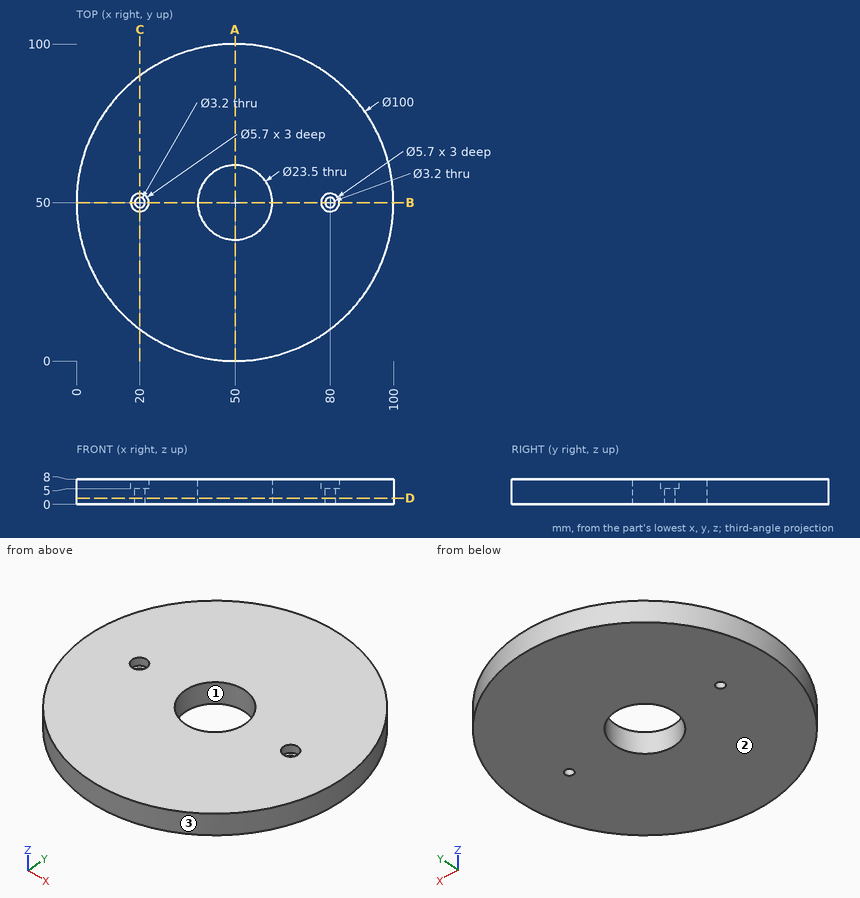
Source: three-view drawing plus pictorial views. Frame: mm from the lowest corner of the part. Coordinates: 2 decimals unless noted, no trailing zeros. Order: outer loops, then holes, each group sorted by start corner. A loop starts at its lowest first (then second) coordinate and runs counter-clockwise, first axis right, second up. Notation, with made-up numbers: M 63,67 L 98,67 A24 ccw 98,100 Z; hole C -6,42 d10. An arc over 180 degrees is marked long. One line per question, with ' | ' between items. Start each with the question number.
Item 1: Cut plane C-C, the plane x = 20. Return the cut outline in (y, z), then the cut area to 3 significant figures.
Item 2: Cut plane B-B, the plane y = 50. Return the cut outline in (x, z).
Item 3: Pin query (flat end, axial travel): pin 1 Ø4 at (y, z) = (66.5, 2) entering from -X; pin 2 Ø1.5 at (y, z) = (70.5, 7) entering from -X; pin 3 Ø3.5 at (x, y) = (80, 50) entering from +Z. Return the tip coordinate at first contact, or that it passes through.
Item 4: Ray query, probe 1 along Y at (x, z) = (50, 6.25); probe 2 along Y at (x, z) = (80, 6.55); probe 3 along X at (y, z) = (74.5, 2.5). Return the intervals inside material, ascending. Write a range as [from, to].
Item 5: Cut plane A-A, the plane x = 50. Return the cut outline in (y, z), then the cut area to 3 significant figures.
Item 6: Draft query along X for the marked faces 1, 2 and 3. Return one class per face: released by +X, released by -X, zero draft, split by the parting line, or undercut.
Item 7: Cut plane D-D, the plane z = 2. Return the cut outline in (x, y), then the cut area to 3 significant figures.
A:
1) outline: M 10,0 L 48.4,0 L 48.4,5 L 47.15,5 L 47.15,8 L 10,8 Z; M 51.6,0 L 90,0 L 90,8 L 52.85,8 L 52.85,5 L 51.6,5 Z | area: 607 mm2
2) outline: M 0,0 L 18.4,0 L 18.4,5 L 17.15,5 L 17.15,8 L 0,8 Z; M 21.6,0 L 38.25,0 L 38.25,8 L 22.85,8 L 22.85,5 L 21.6,5 Z; M 61.75,0 L 78.4,0 L 78.4,5 L 77.15,5 L 77.15,8 L 61.75,8 Z; M 81.6,0 L 100,0 L 100,8 L 82.85,8 L 82.85,5 L 81.6,5 Z
3) pin 1: stops at x = 2.15 | pin 2: stops at x = 4.07 | pin 3: stops at z = 5
4) probe 1: y = [0, 38.25], [61.75, 100] | probe 2: y = [10, 47.15], [52.85, 90] | probe 3: x = [6.41, 93.59]
5) outline: M 0,0 L 38.25,0 L 38.25,8 L 0,8 Z; M 61.75,0 L 100,0 L 100,8 L 61.75,8 Z | area: 612 mm2
6) face 1: undercut | face 2: zero draft | face 3: split by the parting line
7) outline: C 50,50 d100; hole C 20,50 d3.2; hole C 50,50 d23.5; hole C 80,50 d3.2 | area: 7,400 mm2
